Check sheet for the drawn part. Datum: minimum x, y, z corner. Units: mm. Round coordinates to 2 decimals unless told otherwise and drop trailing zeros. Loops run counter-clockwise (first coordinate to the right, second up) from the corner with the lowest first, then second, coordinate; pieces in that order, holes last. Notation, with made-up numbers: (80, -25.75) -> (135, -25.75) arc R23 cw to (135, 9.25) -> close; hole circle Ø5 at (-5, 19). An arc over 180 degrees is marked (long way). Write item = value, one per line. Start each with the question number.
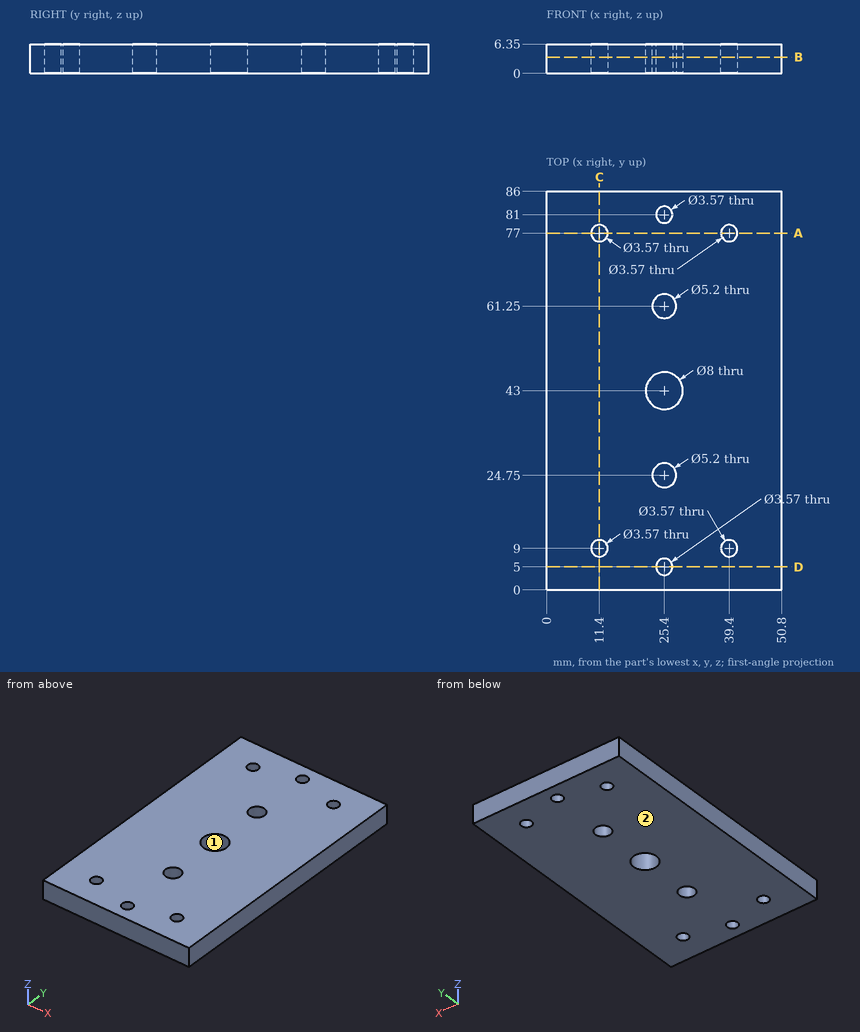
(1) Section check B-B on z = 3.5. Give the number of separate pieces and of enclosed holes in the cut face, then the cut area to 3 significant figures.
(2) Section check C-C on x = 11.4. Enter the section's corners in (y, z) (3 decimals).
(3) Section check A-A on y = 77. Enter the section's corners in (x, z) (3 decimals).
(4) Depth check by flat-ended pin: pin 1 Ø8.5 at (x, y) = (25.4, 61.25) entering from +Z. Enter the tip coordinate at first touch or a pass-through.
(5) Section check D-D on y = 5. Enter the section's corners in (x, z) (3 decimals).
(6) Scan lines: line 1 (Y direction, x = 25.4, z = 2) (3 decimals); line 2 (Y direction, x = 11.4, z = 2.25) (3 decimals); line 3 (Y direction, x = 38.5, z = 3.25). Record each from-to range of solid material in increasing order. Write a range as [from, to].
(7) Draft check along X on the marked faces 1 and 2. Enter one of: +X half, -X half, draft (parallel to the pull), parting line (faces both ways), or undercut.
Computed values:
q1.separate_pieces = 1
q1.enclosed_holes = 9
q1.area = 4,220 mm²
q2.outline = (0, 0) -> (7.215, 0) -> (7.215, 6.35) -> (0, 6.35) -> close; (10.785, 0) -> (75.215, 0) -> (75.215, 6.35) -> (10.785, 6.35) -> close; (78.785, 0) -> (86, 0) -> (86, 6.35) -> (78.785, 6.35) -> close
q3.outline = (0, 0) -> (9.615, 0) -> (9.615, 6.35) -> (0, 6.35) -> close; (13.185, 0) -> (37.615, 0) -> (37.615, 6.35) -> (13.185, 6.35) -> close; (41.185, 0) -> (50.8, 0) -> (50.8, 6.35) -> (41.185, 6.35) -> close
q4.pin_1 = 6.35
q5.outline = (0, 0) -> (23.615, 0) -> (23.615, 6.35) -> (0, 6.35) -> close; (27.185, 0) -> (50.8, 0) -> (50.8, 6.35) -> (27.185, 6.35) -> close
q6.line_1 = [0, 3.215], [6.785, 22.15], [27.35, 39], [47, 58.65], [63.85, 79.215], [82.785, 86]
q6.line_2 = [0, 7.215], [10.785, 75.215], [78.785, 86]
q6.line_3 = [0, 7.46], [10.54, 75.46], [78.54, 86]
q7.face_1 = undercut
q7.face_2 = draft
